The drawing under review shows one solid part. Ordinate dimensions are in mm from its lowest x, y, z. A direction names the side the tool comes from. Coordinates: 2 decimals unless noted, no trailing zeros. Write each loop counter-clockwise with the first axis right and the second up, starting at its lowest first coordinate (ties: lowest second). Pieces come first, ordered by that corner, then holes.
Q1. Add section B-B, the plane y = 39.5. Give the boundary of the cut face in (x, z) (1 decimal).
Q2. Add section D-D, the plane z = 29. Give the boundary of the cut face in (x, y) (1 decimal).
Q3. Add section A-A, the plane z = 88.9. Give the boundary of the cut face in (x, y) (1 decimal).
Q4. Machinability: for the marked faces 1 and 2, which of the approach directions +Z, -Z, +X, -X, +Y, -Y give a long, thin tool a straight path to every point of the face, cutting with its end or side? Answer none if there is none.
Q5. Clearance check with flat-ended pins moving along their axes: pin 1 Ø4.5 at (y, z) = (25.4, 12.7) entering from -X (3 decimals); pin 2 Ø1.5 at (y, z) = (14.5, 11.5) entering from +X (3 decimals); pin 3 Ø5.5 at (x, z) = (25.4, 63.5) entering from +Y (3 decimals). State where each tip first meets the part, or that it passes through.
Q6. To check wall thickness, follow probe 1 along Y at (x, z) = (2, 38); probe 2 along Z at (x, y) = (38.1, 0.8); probe 3 along X at (y, z) = (16.5, 26.5) (1 decimal). State the ranges of each line that lie inside material, in increasing order.
Q7. Add section C-C, the plane x = 37.5. Give the boundary of the cut face in (y, z) (1 decimal), plus the area to 3 significant figures.
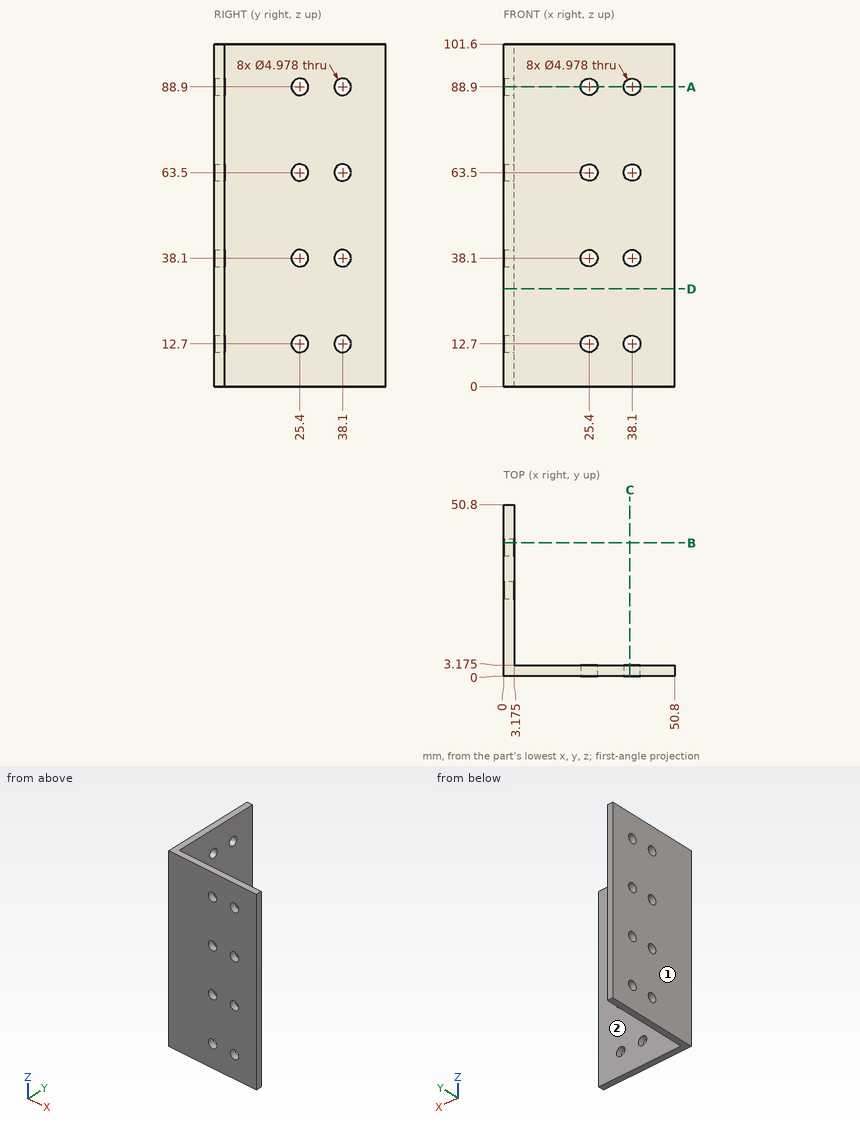
Here are the results:
1. outline: (0, 0) - (3.2, 0) - (3.2, 10.6) - (0, 10.6) - close; (0, 14.8) - (3.2, 14.8) - (3.2, 36) - (0, 36) - close; (0, 40.2) - (3.2, 40.2) - (3.2, 61.4) - (0, 61.4) - close; (0, 65.6) - (3.2, 65.6) - (3.2, 86.8) - (0, 86.8) - close; (0, 91) - (3.2, 91) - (3.2, 101.6) - (0, 101.6) - close
2. outline: (0, 0) - (50.8, 0) - (50.8, 3.2) - (3.2, 3.2) - (3.2, 50.8) - (0, 50.8) - close
3. outline: (0, 0) - (22.9, 0) - (22.9, 3.2) - (3.2, 3.2) - (3.2, 22.9) - (0, 22.9) - close; (0, 27.9) - (3.2, 27.9) - (3.2, 35.6) - (0, 35.6) - close; (0, 40.6) - (3.2, 40.6) - (3.2, 50.8) - (0, 50.8) - close; (27.9, 0) - (35.6, 0) - (35.6, 3.2) - (27.9, 3.2) - close; (40.6, 0) - (50.8, 0) - (50.8, 3.2) - (40.6, 3.2) - close
4. face 1: +Z, -Z, -X, +Y, -Y
4. face 2: +Z, -Z, +X, +Y
5. pin 1: passes through
5. pin 2: stops at x = 3.175
5. pin 3: stops at y = 3.175
6. probe 1: y = 0 to 22.91, 27.89 to 35.61, 40.59 to 50.8
6. probe 2: z = 0 to 10.21, 15.19 to 35.61, 40.59 to 61.01, 65.99 to 86.41, 91.39 to 101.6
6. probe 3: x = 0 to 3.2
7. outline: (0, 0) - (3.2, 0) - (3.2, 10.3) - (0, 10.3) - close; (0, 15.1) - (3.2, 15.1) - (3.2, 35.7) - (0, 35.7) - close; (0, 40.5) - (3.2, 40.5) - (3.2, 61.1) - (0, 61.1) - close; (0, 65.9) - (3.2, 65.9) - (3.2, 86.5) - (0, 86.5) - close; (0, 91.3) - (3.2, 91.3) - (3.2, 101.6) - (0, 101.6) - close
7. area: 261 mm2
